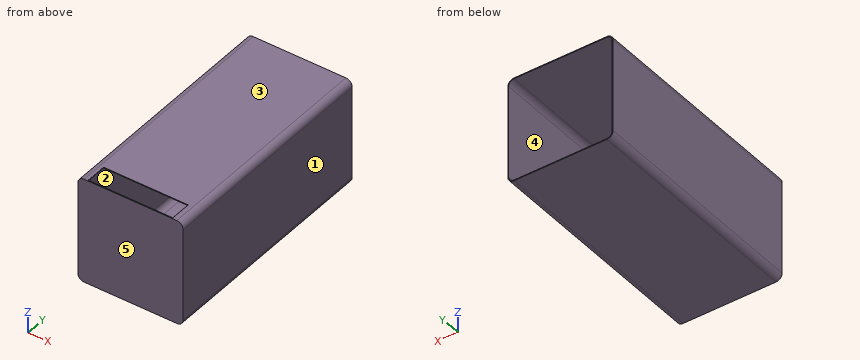
from build123d import *

# Parameters (mm, degrees)
EXTRUDE_1_DEPTH = 5
EXTRUDE_2_DEPTH = 100
EXTRUDE_3_DEPTH = 1000


with BuildPart() as part:
    # 草图1 → 凸台-拉伸1 (new body)
    with BuildSketch(Plane(origin=(0, 0, 0), x_dir=(1, 0, 0), z_dir=(0, 1, 0))):
        with BuildLine():
            Line((220, 250), (-220, 250))
            ThreePointArc((-220, 250), (-241.213203436, 241.213203436), (-250, 220))
            Line((-250, 220), (-250, -220))
            ThreePointArc((-250, -220), (-241.213203436, -241.213203436), (-220, -250))
            Line((-220, -250), (220, -250))
            ThreePointArc((220, -250), (241.213203436, -241.213203436), (250, -220))
            Line((250, -220), (250, 220))
            ThreePointArc((250, 220), (241.213203436, 241.213203436), (220, 250))
        make_face()
    extrude(amount=EXTRUDE_1_DEPTH)

    # 草图2 → 凸台-拉伸2 (add)
    with BuildSketch(Plane(origin=(0, 5, 0), x_dir=(1, 0, 0), z_dir=(0, 1, 0))):
        with BuildLine():
            Line((-220, -246), (-204.515980858, -246))
            ThreePointArc((-204.515980858, -246), (-203.455320686, -246.439339828), (-203.015980858, -247.5))
            Line((-203.015980858, -247.5), (-203.015980858, -248.5))
            ThreePointArc((-203.015980858, -248.5), (-203.455320686, -249.560660172), (-204.515980858, -250))
            Line((-204.515980858, -250), (-220, -250))
            ThreePointArc((-220, -250), (-241.213203436, -241.213203436), (-250, -220))
            Line((-250, -220), (-250, 220))
            ThreePointArc((-250, 220), (-241.213203436, 241.213203436), (-220, 250))
            Line((-220, 250), (220, 250))
            ThreePointArc((220, 250), (241.213203436, 241.213203436), (250, 220))
            Line((250, 220), (250, -220))
            ThreePointArc((250, -220), (241.213203436, -241.213203436), (220, -250))
            Line((220, -250), (198.484019142, -250))
            ThreePointArc((198.484019142, -250), (197.42335897, -249.560660172), (196.984019142, -248.5))
            Line((196.984019142, -248.5), (196.984019142, -247.5))
            ThreePointArc((196.984019142, -247.5), (197.42335897, -246.439339828), (198.484019142, -246))
            Line((198.484019142, -246), (220, -246))
            ThreePointArc((220, -246), (238.384776311, -238.384776311), (246, -220))
            Line((246, -220), (246, 220))
            ThreePointArc((246, 220), (238.384776311, 238.384776311), (220, 246))
            Line((220, 246), (-220, 246))
            ThreePointArc((-220, 246), (-238.384776311, 238.384776311), (-246, 220))
            Line((-246, 220), (-246, -220))
            ThreePointArc((-246, -220), (-238.384776311, -238.384776311), (-220, -246))
        make_face()
    extrude(amount=EXTRUDE_2_DEPTH)

    # 草图3 → 凸台-拉伸3 (add)
    with BuildSketch(Plane(origin=(0, 105, 0), x_dir=(1, 0, 0), z_dir=(0, 1, 0))):
        with BuildLine():
            Line((-204.515980858, -246), (-220, -246))
            ThreePointArc((-220, -246), (-238.384776311, -238.384776311), (-246, -220))
            Line((-246, -220), (-246, 220))
            ThreePointArc((-246, 220), (-238.384776311, 238.384776311), (-220, 246))
            Line((-220, 246), (220, 246))
            ThreePointArc((220, 246), (238.384776311, 238.384776311), (246, 220))
            Line((246, 220), (246, -220))
            ThreePointArc((246, -220), (238.384776311, -238.384776311), (220, -246))
            Line((220, -246), (198.484019142, -246))
            ThreePointArc((198.484019142, -246), (197.42335897, -246.439339828), (196.984019142, -247.5))
            Line((196.984019142, -247.5), (196.984019142, -248.5))
            ThreePointArc((196.984019142, -248.5), (197.42335897, -249.560660172), (198.484019142, -250))
            Line((198.484019142, -250), (220, -250))
            ThreePointArc((220, -250), (241.213203436, -241.213203436), (250, -220))
            Line((250, -220), (250, 220))
            ThreePointArc((250, 220), (241.213203436, 241.213203436), (220, 250))
            Line((220, 250), (-220, 250))
            ThreePointArc((-220, 250), (-241.213203436, 241.213203436), (-250, 220))
            Line((-250, 220), (-250, -220))
            ThreePointArc((-250, -220), (-241.213203436, -241.213203436), (-220, -250))
            Line((-220, -250), (-204.515980858, -250))
            ThreePointArc((-204.515980858, -250), (-203.455320686, -249.560660172), (-203.015980858, -248.5))
            Line((-203.015980858, -248.5), (-203.015980858, -247.5))
            ThreePointArc((-203.015980858, -247.5), (-203.455320686, -246.439339828), (-204.515980858, -246))
        make_face()
        with BuildLine():
            Line((-204.515980858, -250), (198.484019142, -250))
            ThreePointArc((198.484019142, -250), (197.42335897, -249.560660172), (196.984019142, -248.5))
            Line((196.984019142, -248.5), (196.984019142, -247.5))
            ThreePointArc((196.984019142, -247.5), (197.42335897, -246.439339828), (198.484019142, -246))
            Line((198.484019142, -246), (-204.515980858, -246))
            ThreePointArc((-204.515980858, -246), (-203.455320686, -246.439339828), (-203.015980858, -247.5))
            Line((-203.015980858, -247.5), (-203.015980858, -248.5))
            ThreePointArc((-203.015980858, -248.5), (-203.455320686, -249.560660172), (-204.515980858, -250))
        make_face()
    extrude(amount=EXTRUDE_3_DEPTH)


solid = part.part
The listing builds one solid part. Answer for the finished solid, in the listing's coordinates (mm). Face numbers are marked on the shaded views. A direction names the side the tool comes from. Round coordinates to 2 decimals unless told otherwise and drop trailing zeros. Order: outer loops, then holes, each group sorted by start corner. A loop starts at its lowest first (then second) coordinate and runs counter-clockwise, first axis right, second up. Notation, with made-up numbers: (78.5, 33.5) -> (125.5, 33.5) arc R14 cw to (125.5, 39.5) -> close; hole circle Ø9 at (48.5, 36.5). An arc over 180 degrees is marked (long way). Put each result on its own line as item: value.
Q1. Section A-A, the plane x = 139.5 is taken. Write down the section's boundary in (y, z).
Results list:
outline: (0, -250) -> (1105, -250) -> (1105, -246) -> (5, -246) -> (5, 250) -> (0, 250) -> close; (105, 246) -> (1105, 246) -> (1105, 250) -> (105, 250) -> close
Q2. Consider line 1 along X through (y, z) = (368.5, 21.5); line 2 along Y through (x, z) = (-172, 82). Determine where each line is inside the solid, lowest interval first.
Results list:
line 1: -250 to -246, 246 to 250
line 2: 0 to 5
Q3. Section C-C, the plane z = -192 is taken. Write down the section's boundary in (x, y), and give its area (3 significant figures).
Results list:
outline: (-250, 0) -> (250, 0) -> (250, 1105) -> (246, 1105) -> (246, 5) -> (-246, 5) -> (-246, 1105) -> (-250, 1105) -> close
area: 11,300 mm^2
Q4. Which of the six approach directions +Z, -Z, +X, -X, +Y, -Y give full straight-line access (tool end or side, diameter ignored) to the marked faces 4 and 5?
Results list:
face 4: +Y
face 5: +Z, -Z, +X, -X, -Y
Q5. Section B-B, the plane y = 933 is taken. Write down the section's boundary in (x, z).
Results list:
outline: (-250, -220) arc R30 ccw to (-220, -250) -> (220, -250) arc R30 ccw to (250, -220) -> (250, 220) arc R30 ccw to (220, 250) -> (-220, 250) arc R30 ccw to (-250, 220) -> close; hole (-246, -220) arc R26 ccw to (-220, -246) -> (220, -246) arc R26 ccw to (246, -220) -> (246, 220) arc R26 ccw to (220, 246) -> (-220, 246) arc R26 ccw to (-246, 220) -> close
Q6. Determine the mould class of the marked faces 1, 2 and 3 for opening direction Z: pulls with the +Z half, pulls with the -Z half, needs draft (parallel to the pull), parting line crosses it, or undercut.
Results list:
face 1: needs draft
face 2: undercut
face 3: pulls with the +Z half
Q7. Each of these flat-tipped pins is pushed along its axis until it touches: P1, Ø0.8, axis at y = 43.5, z = 248, coming from the -X side; P2, Ø0.5, axis at y = 64, z = 248, coming from the +X side. Where does it stop, or does it pass through?
Results list:
P1: x = -231.76
P2: x = 231.4
